from build123d import *

# Parameters (mm, degrees)
SKETCH1_W           = 420
SKETCH1_H           = 420
BOSS_EXTRUDE1_DEPTH = 6
SKETCH3_W           = 6
SKETCH3_H           = 60
SKETCH3_W_2         = 60
SKETCH3_H_2         = 6
CUT_EXTRUDE2_DEPTH  = 7
CUT_EXTRUDE3_DEPTH  = 7


with BuildPart() as part:
    # Sketch1 → Boss-Extrude1 (new body)
    with BuildSketch(Plane(origin=(0, 0, 0), x_dir=(1, 0, 0), z_dir=(0, 1, 0))):
        Rectangle(SKETCH1_W, SKETCH1_H)
    extrude(amount=BOSS_EXTRUDE1_DEPTH)

    # Sketch3 → Cut-Extrude2 (cut, through all)
    with BuildSketch(Plane(origin=(0, 6, 0), x_dir=(1, 0, 0), z_dir=(0, 1, 0))):
        with Locations((-207, 120)):
            Rectangle(SKETCH3_W, SKETCH3_H)
        with Locations((-207, 0)):
            Rectangle(SKETCH3_W, SKETCH3_H)
        with Locations((-207, -120)):
            Rectangle(SKETCH3_W, SKETCH3_H)
        with Locations((120, 207)):
            Rectangle(SKETCH3_W_2, SKETCH3_H_2)
        with Locations((0, 207)):
            Rectangle(SKETCH3_W_2, SKETCH3_H_2)
        with Locations((-120, 207)):
            Rectangle(SKETCH3_W_2, SKETCH3_H_2)
        with Locations((207, -120)):
            Rectangle(SKETCH3_W, SKETCH3_H)
        with Locations((207, 0)):
            Rectangle(SKETCH3_W, SKETCH3_H)
        with Locations((207, 120)):
            Rectangle(SKETCH3_W, SKETCH3_H)
        with Locations((-120, -207)):
            Rectangle(SKETCH3_W_2, SKETCH3_H_2)
        with Locations((0, -207)):
            Rectangle(SKETCH3_W_2, SKETCH3_H_2)
        with Locations((120, -207)):
            Rectangle(SKETCH3_W_2, SKETCH3_H_2)
    extrude(amount=-CUT_EXTRUDE2_DEPTH, mode=Mode.SUBTRACT)

    # Sketch5 → Cut-Extrude3 (cut, through all)
    with BuildSketch(Plane(origin=(0, 6, 0), x_dir=(1, 0, 0), z_dir=(0, 1, 0))):
        Polygon((3, 3), (15, 3), (15, -3), (3, -3), (3, -15), (-3, -15), (-3, -3), (-15, -3), (-15, 3), (-3, 3), (-3, 15), (3, 15), align=None)
    extrude(amount=-CUT_EXTRUDE3_DEPTH, mode=Mode.SUBTRACT)


solid = part.part
For this review, take the finished solid that the model builds, in its own axes (mm). Round coordinates to 2 decimals unless told otherwise and drop trailing zeros. Loops run counter-clockwise (first coordinate to the right, second up) from the corner with the lowest first, then second, coordinate; pieces in that order, holes last. Notation, with made-up numbers: (26, 59) - (40, 59) arc R8 cw to (40, 66) - close; hole circle Ø10 at (73.25, -1). An arc over 180 degrees is marked (long way). Use one line per item in the form item = value.
1) We need section B-B on x = 101. Write out the cut boundary in (y, z).
Solutions:
outline = (0, -204) - (6, -204) - (6, 204) - (0, 204) - close
2) Wall thickness on probe 1 along Z at (x, y) = (-14.5, 2.65); probe 2 along Z at (x, y) = (-131, 2.1): over which ranges is each line inside the solid? List them lowest first.
Solutions:
probe_1 = -204 to -3, 3 to 204
probe_2 = -204 to 204
3) We need section A-A on x = -9. Write out the cut boundary in (y, z), then the cut area to 3 significant figures.
Solutions:
outline = (0, -204) - (6, -204) - (6, -3) - (0, -3) - close; (0, 3) - (6, 3) - (6, 204) - (0, 204) - close
area = 2,410 mm2
4) We need section C-C on z = -105. Write out the cut boundary in (x, y).
Solutions:
outline = (-204, 0) - (204, 0) - (204, 6) - (-204, 6) - close
5) Clearance check with flat-ended pins moving along their axes: P1, Ø3, axis at x = 112, y = 2.5, coming from the -Z side; P2, Ø3, axis at y = 1.5, z = 0, coming from the +X side; P3, Ø3, axis at y = 2, z = -11, coming from the -X side. State where each tip first meets the part, or that it passes through.
Solutions:
P1 = -204
P2 = 204
P3 = -204
